from build123d import *

# Parameters (mm, degrees)
CROQUIS1_W                 = 53
CROQUIS1_H                 = 4
CHAFL_N1_SIZE              = 1
CORTAR_EXTRUIR1_DEPTH      = 29.814059068
CORTAR_EXTRUIR1_DEPTH_BACK = 29.814059068
CROQUIS2_W                 = 45.5
CROQUIS2_H                 = 2.5


with BuildPart() as part:
    # Croquis1 → Revolución1 (revolve)
    with BuildSketch(Plane(origin=(0, 0, 0), x_dir=(0, 0, -1), z_dir=(1, 0, 0)), mode=Mode.PRIVATE) as revoluci_n1_sk:
        with Locations((0, 6)):
            Rectangle(CROQUIS1_W, CROQUIS1_H)
    revolve(revoluci_n1_sk.sketch.rotate(Axis((0, 0, 35.899159664), (0, 0, -1)), 90), axis=Axis((0, 0, 35.899159664), (0, 0, -1)))

    # Chaflán1
    chafl_n1_edges = [part.edges().sort_by_distance(p)[0] for p in [
        (-4, 0, 26.5),
    ]]
    chamfer(chafl_n1_edges, length=CHAFL_N1_SIZE)

    # Croquis2 → Cortar-Extruir1 (cut, two sides: drawn at the far end of the back side and taken through both)
    with BuildSketch(Plane(origin=(0, 0, 0), x_dir=(0, 0, -1), z_dir=(1, 0, 0)).offset(-CORTAR_EXTRUIR1_DEPTH_BACK)):
        with Locations((-1.25, 6.75)):
            Rectangle(CROQUIS2_W, CROQUIS2_H)
    extrude(amount=CORTAR_EXTRUIR1_DEPTH + CORTAR_EXTRUIR1_DEPTH_BACK, mode=Mode.SUBTRACT)


solid = part.part
Part model, mm, in its own coordinate system. A direction names the side the tool comes from. Give positions to 0.01 mm unless a question says otherwise; leave off trailing zeros. Order: outer loops, then holes, each group sorted by start corner. A loop starts at its lowest first (then second) coordinate and runs counter-clockwise, first axis right, second up. Notation, with made-up numbers: (-21.5, -14.5) -> (-11.5, -14.5) arc R26 cw to (-11.5, 19.5) -> close; hole circle Ø3 at (-20.5, 66.25). An arc over 180 degrees is marked (long way). Use one line per item in the form item = value.
(1) Flat gauge pins, fed straight in: P1, Ø4, axis at y = 5, z = -20.5, coming from the -X side; P2, Ø2, axis at x = -5, z = -9, coming from the -Y side; P3, Ø1, axis at x = 3.5, z = -4, coming from the -Y side. Where does each tip first touch, or does it go through?
Solution:
P1 = -7.42
P2 = -6.93
P3 = -7.42
(2) Tool access for faces 1 (the face through (0, 6, -21.5)), 2 (the face through (-5.2, -0.1, 26.5)): list every direction of +Z, -Z, +X, -X, +Y, -Y with a clear straight run to the whole face (end or side of a thin tool).
Solution:
face_1 = +X, -X, +Y
face_2 = +Z, +X, -X, +Y, -Y
(3) Pull direction X, two halves, no side cores. Call faces 3 (the face through (-0.867, 3.905, -0.864)), 4 (the face through (-1.041, -7.932, -0.371)), 5 (the face through (0, 5.5, 2)): +X half, -X half, draft (parallel to the pull), parting line (faces both ways), or undercut.
Solution:
face_3 = undercut
face_4 = parting line
face_5 = draft
(4) Saw through at A-A (x = 0). Write the cut outline in (y, z).
Solution:
outline = (-8, -26.5) -> (-4, -26.5) -> (-4, 25.5) -> (-5, 26.5) -> (-8, 26.5) -> close; (4, -26.5) -> (8, -26.5) -> (8, -21.5) -> (5.5, -21.5) -> (5.5, 24) -> (8, 24) -> (8, 26.5) -> (5, 26.5) -> (4, 25.5) -> close
(5) Saw through at B-B (y = 0). Write the cut outline in (x, z), then the cut area to 3 significant figures.
Solution:
outline = (-8, -26.5) -> (-4, -26.5) -> (-4, 25.5) -> (-5, 26.5) -> (-8, 26.5) -> close; (4, -26.5) -> (8, -26.5) -> (8, 26.5) -> (5, 26.5) -> (4, 25.5) -> close
area = 423 mm²
(6) Saw through at D-D (x = -6.5). Write the cut outline in (y, z), then the cut area to 3 significant figures.
Solution:
outline = (-4.66, -26.5) -> (4.66, -26.5) -> (4.66, 26.5) -> (-4.66, 26.5) -> close
area = 494 mm²
(7) Drill centre lines: line 1 (Y direction, x = 0, z = -11); line 2 (Z direction, x = -2, y = 6.75); line 3 (Y direction, x = -1.25, z = -18.5). Where is each one in solid material? Low to high. Write a range as from..to.
Solution:
line_1 = -8..-4, 4..5.5
line_2 = -26.5..-21.5, 24..26.5
line_3 = -7.9..-3.8, 3.8..5.5
(8) Saw through at C-C (z = -21). Write the cut outline in (x, y), then the cut area to 3 significant figures.
Solution:
outline = (-5.81, 5.5) arc R8 ccw (long way) to (5.81, 5.5) -> close; hole circle Ø8 at (0, 0)
area = 131 mm²
